Geometry: see drawing. Coordinates: mm, zero at the bounding-box minimum. A direction names the side the tool comes from. Give positions to 0.01 mm unless a question says otherwise; leave off trailing zeros. Loops run counter-clockwise (first coordinate to the right, second up) from the corner with the lowest first, then second, coordinate; pieces in that order, holes last. Notation, with made-up numbers: M 14,-8.75 L 30,-8.75 A13 cw 30,8.25 Z; hole C 28.25,-4.75 d10. An arc over 180 degrees is marked long. Put each result on its own line as item: value.
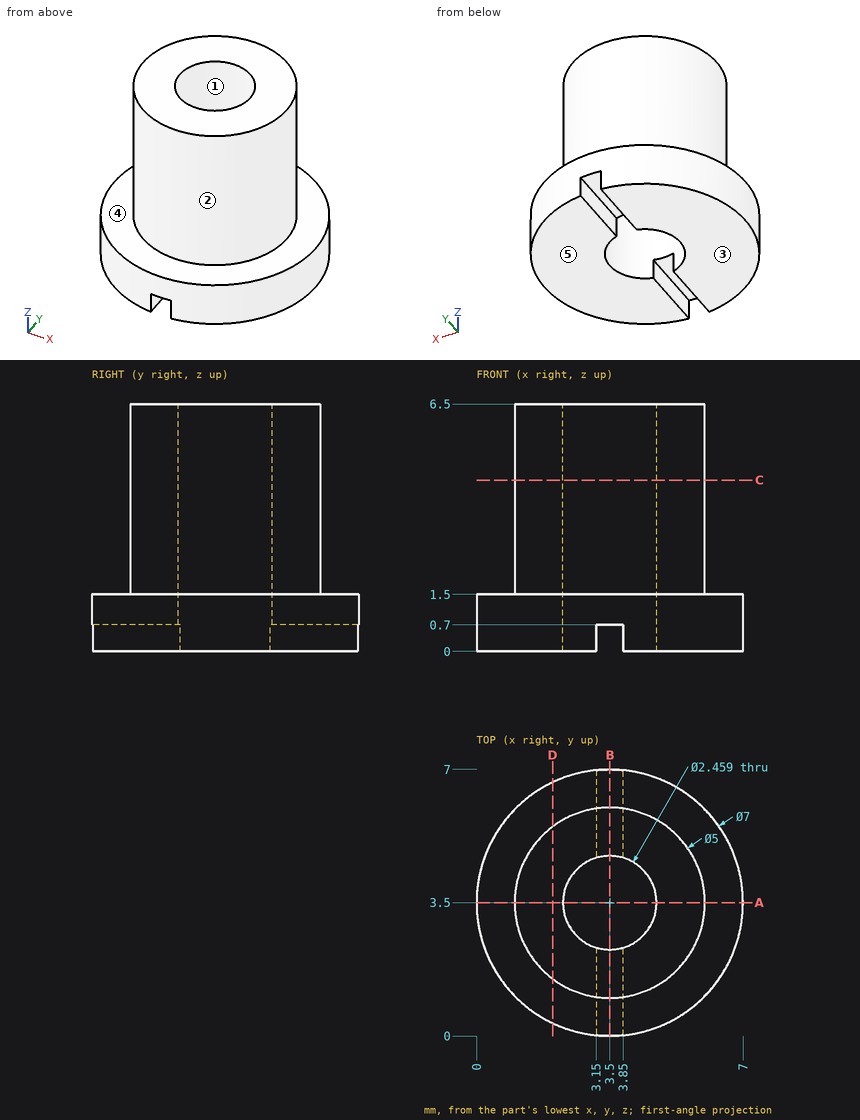
Item 1: Section A-A on y = 3.5. Output: boundary loops of the cut face in (x, z), then the cut area to 3 significant figures.
Output values:
outline: M 0,0 L 2.27,0 L 2.27,6.5 L 1,6.5 L 1,1.5 L 0,1.5 Z; M 4.73,0 L 7,0 L 7,1.5 L 6,1.5 L 6,6.5 L 4.73,6.5 Z
area: 19.5 mm²
Item 2: Section B-B on x = 3.5. Output: boundary loops of the cut face in (y, z), then the cut area to 3 significant figures.
Output values:
outline: M 0,0.7 L 2.27,0.7 L 2.27,6.5 L 1,6.5 L 1,1.5 L 0,1.5 Z; M 4.73,0.7 L 7,0.7 L 7,1.5 L 6,1.5 L 6,6.5 L 4.73,6.5 Z
area: 16.3 mm²
Item 3: Pin query (flat end, axial travel): pin 1 Ø0.6 at (y, z) = (5.5, 0) entering from -X; pin 2 Ø0.8 at (y, z) = (0.5, 0.5) entering from +X; pin 3 Ø2 at (y, z) = (2.5, 3.5) entering from +X. Return the tip coordinate at first contact, or that it passes through.
Output values:
pin 1: x = 0.44
pin 2: x = 5.84
pin 3: x = 6
Item 4: Set-up query: the marked faces 4 and 5. Return all of +Z, -Z, +X, -X, +Y, -Y with unobstructed straight access to the full face (end or side cutting, diameter ignored); none if empty.
Output values:
face 4: +Z
face 5: -Z, +X, -X, +Y, -Y
Item 5: Mould query, pull axis X, two halves, no side actions, for the marked faces 1, 2 and 3. Classes: pulls with the +X half, pulls with the -X half, needs draft (parallel to the pull), parting line crosses it, or undercut.
Output values:
face 1: undercut
face 2: parting line crosses it
face 3: needs draft
Item 6: Line query: probe 1 along Y at (x, z) = (3.5, 2); probe 2 along Z at (x, y) = (3.25, 2); probe 3 along Z at (x, y) = (0.75, 4.5). Output: solid intervals per line, ascending. Write a range as [from, to].
Output values:
probe 1: [1, 2.27], [4.73, 6]
probe 2: [0.7, 6.5]
probe 3: [0, 1.5]
Item 7: Section C-C on z = 4.5. Output: boundary loops of the cut face in (x, y), then the cut area to 3 significant figures.
Output values:
outline: C 3.5,3.5 d5; hole C 3.5,3.5 d2.46
area: 14.9 mm²
Item 8: Section D-D on x = 2. Output: boundary loops of the cut face in (y, z).
Output values:
outline: M 0.34,0 L 6.66,0 L 6.66,1.5 L 5.5,1.5 L 5.5,6.5 L 1.5,6.5 L 1.5,1.5 L 0.34,1.5 Z
